Geometry check sheet. Reference: the model listing, model coordinates, mm. A direction names the side the tool comes from. Give positions to 0.01 mm unless a question says otherwise; leave off trailing zeros. Write each loop counter-clockwise with the first axis right and the second up, starting at its lowest first coordinate (ties: lowest second). Pieces come first, ordered by that corner, then holes. Notation, with made-up numbers: M 61.25,-34 L 118.25,-34 A12 ccw 118.25,-11 Z; hole C 32,60.25 d9. An arc over 180 degrees is marked long. One line per item, written item: value. Start each with the question number.
1. Scan lines: line 1 (X direction, y = 2.35, z = -4); line 2 (X direction, y = 2.6, z = -12); line 3 (X direction, y = 0.7, z = -10). Record each from-to range of solid material in increasing order.
2. Cross-section at B-B on x = 7.75. Record the cut outline in (y, z), then the cut area to 3 significant figures.
3. Cross-section at C-C on z = -12. Record the cut outline in (x, y).
4. Cross-section at A-A on y = 2.85. Record the cut outline in (x, z).
5. Tool access check on faces 5 (the face through (6.4, 1, -10)), 6 (the face through (4, 2, -16)), 7 (the face through (9.976, 3.989, -5.29)). Record the directions out of +Z, -Z, +X, -X, +Y, -Y that give a thin tool (end or side, any length) a straight path to the whole face; none if there is none.
6. Cross-section at D-D on y = 3.9. Record the cut outline in (x, z).
7. Gauge pin test, flat ends, axial feed: pin 1 (1 mm diameter, centred on x = 10, y = 1.5, fed in from -Z); pin 2 (1.3 mm diameter, centred on x = 4, z = -12.5, fed in from -Y). Record the tip position at first contact, or that the pin passes through.
8. Release check for a two-part mould opening along X. For faces 1 (the face through (1.6, 1, -8)), 2 (the face through (16, 2, -4)), 3 (the face through (0, 2, -8)), 4 (the face through (4, 3.2, -4)) record: pulls with the +X half, pulls with the -X half, needs draft (parallel to the pull), parting line crosses it, or undercut.
from build123d import *

# Parameters (mm, degrees)
BOSS_EXTRUDE1_DEPTH = 3.2
SKETCH2_R           = 2.4
BOSS_EXTRUDE2_DEPTH = 1.6
SHELL1_T            = -1.6


with BuildPart() as part:
    # Sketch1 → Boss-Extrude1 (new body)
    with BuildSketch(Plane(origin=(0, 0, 0), x_dir=(1, 0, 0), z_dir=(0, 1, 0))):
        Polygon((0, 0), (0, 16), (8, 16), (8, 8), (16, 8), (16, 0), align=None)
    extrude(amount=BOSS_EXTRUDE1_DEPTH)

    # Sketch2 → Boss-Extrude2 (add)
    with BuildSketch(Plane(origin=(0, 3.2, 0), x_dir=(1, 0, 0), z_dir=(0, 1, 0))):
        with Locations(Location((4, 4, 0), (0, 0, 90))):
            Circle(SKETCH2_R)
        with Locations(Location((4, 12, 0), (0, 0, 90))):
            Circle(SKETCH2_R)
        with Locations(Location((12, 4, 0), (0, 0, 90))):
            Circle(SKETCH2_R)
    extrude(amount=BOSS_EXTRUDE2_DEPTH)

    # Shell1
    shell1_openings = [part.faces().sort_by_distance(p)[0] for p in [
        (6.666666667, 0, -6.666666667),
    ]]
    offset(amount=SHELL1_T, openings=shell1_openings, kind=Kind.INTERSECTION)


solid = part.part
Report:
1. line 1: x = 0 to 3.2, 4.8 to 11.2, 12.8 to 16
1. line 2: x = 0 to 3.2, 4.8 to 8
1. line 3: x = 0 to 1.6, 6.4 to 8
2. outline: M 0,-16 L 3.2,-16 L 3.2,0 L 0,0 L 0,-1.6 L 1.6,-1.6 L 1.6,-6.4 L 0,-6.4 Z
2. area: 43.5 mm^2
3. outline: M 0,0 L 1.6,0 L 1.6,1.6 L 3.2,1.6 L 3.2,3.2 L 4.8,3.2 L 4.8,1.6 L 6.4,1.6 L 6.4,0 L 8,0 L 8,3.2 L 6.4,3.2 L 6.4,4.8 L 1.6,4.8 L 1.6,3.2 L 0,3.2 Z
4. outline: M 0,-16 L 8,-16 L 8,-8 L 16,-8 L 16,0 L 0,0 Z; hole C 4,-12 d1.6; hole C 4,-4 d1.6; hole C 12,-4 d1.6
5. face 5: -Y
5. face 6: -Z, +X, -X, +Y, -Y
5. face 7: +Y
6. outline: C 4,-12 d4.8; C 4,-4 d4.8; C 12,-4 d4.8
7. pin 1: stops at z = -8
7. pin 2: stops at y = 1.6
8. face 1: undercut
8. face 2: pulls with the +X half
8. face 3: pulls with the -X half
8. face 4: undercut
